Part model, mm, in its own coordinate system. A direction names the side the tool comes from. Give positions to 0.01 mm unless a question says otherwise; leave off trailing zeros. Write each loop counter-clockwise with the first axis right and the second up, starting at its lowest first coordinate (ties: lowest second). Pieces come first, ordered by that corner, then holes. Notation, with made-up numbers: M 21.5,26 L 61.5,26 A28 ccw 61.5,59 Z; hole C 75,-28.75 d4. An arc over 180 degrees is marked long. Use CSV: the item, a comma, the result in double quotes. Start each with the question number.
1. Band-saw the part on C-C, the plane z = 0.2. Count the separate pieces of the cut face and the enclosed holes in it, then the cut area to 3 significant figures.
2. 3-axis set-ups, long thin cutter, end or side, ignore diameter. For faces 1 (the face through (388.624, -9.204, -0.021)), 2 (the face through (-388.974, -8.598, -0.021)), 3 (the face through (-216.72, -306.95, -0.02)): which of +Z, -Z, +X, -X, +Y, -Y reach the whole face in a straight line?
3. Band-saw the part on B-B, the plane y = 27. List the corners of the cut face in (x, z).
4. Band-saw the part on A-A, the plane x = -63.5. List the corners of the cut face in (y, z), then the cut area to 3 significant figures.
5. Mould opens along Y. For faces 4 (the face through (216.31, -307.66, -0.02)), 5 (the face through (-378.7, 54.89, -0.02)), 6 (the face through (-324.137, 149.399, -0.021)) say: pulls with the +Y half, pulls with the -Y half, needs draft (parallel to the pull), parting line crosses it, or undercut.
6. Drill centre lines: line 1 along X through (y, z) = (112, 1.3); line 2 along X through (y, z) = (-54.5, 0.55); line 3 along Y through (x, z) = (7.5, -0.55). Where is each one in solid material? Low to high. Write a range as from..to.
7. Drop flat-ended pins along their axis: pin 1 Ø1 at (x, z) = (103.5, 1) entering from -Y; pin 2 Ø1.5 at (y, z) = (-341.5, 0) entering from +X; pin 3 Ø8 at (x, y) = (-379.31, -43.84) entering from -Z; pin 4 Ø1.5 at (y, z) = (-126, 1) entering from +X. Give the stop position or say it passes through.
from build123d import *

# Parameters (mm, degrees)
SKETCH_1_R              = 3
EXTRUDE_1_DEPTH         = 1.5
SHEET_START             = -1.5
SHEET_METAL_1_OUTLINE_R = 3
SHEET_METAL_1_DEPTH     = 1.5


# Read off the part's stored shape, not the designer's step: Преобразовать-Твердое тело1
with BuildPart() as part:
    # Sketch 1 → Бобышка-Вытянуть1 (new body)
    with BuildSketch(Plane.XY):
        with BuildLine():
            Line((201.732050808, -332.910161514), (231.299038106, -281.698637287))
            Line((231.299038106, -281.698637287), (247.320508076, -290.948637287))
            Line((247.320508076, -290.948637287), (257.320508076, -273.628129211))
            Line((257.320508076, -273.628129211), (241.299038106, -264.378129211))
            Line((241.299038106, -264.378129211), (366.299038106, -47.871778265))
            Line((366.299038106, -47.871778265), (382.320508076, -57.121778265))
            Line((382.320508076, -57.121778265), (392.320508076, -39.801270189))
            Line((392.320508076, -39.801270189), (376.299038106, -30.551270189))
            Line((376.299038106, -30.551270189), (401.299038106, 12.75))
            ThreePointArc((401.299038106, 12.75), (401.700961894, 14.25), (401.299038106, 15.75))
            Line((401.299038106, 15.75), (356.732050808, 92.942286341))
            Line((356.732050808, 92.942286341), (374.052558883, 102.942286341))
            Line((374.052558883, 102.942286341), (364.052558883, 120.262794416))
            Line((364.052558883, 120.262794416), (346.732050808, 110.262794416))
            Line((346.732050808, 110.262794416), (302.165063509, 187.455080757))
            Line((302.165063509, 187.455080757), (-302.165063509, 187.455080757))
            Line((-302.165063509, 187.455080757), (-346.732050808, 110.262794416))
            Line((-346.732050808, 110.262794416), (-364.052558883, 120.262794416))
            Line((-364.052558883, 120.262794416), (-374.052558883, 102.942286341))
            Line((-374.052558883, 102.942286341), (-356.732050808, 92.942286341))
            Line((-356.732050808, 92.942286341), (-401.299038106, 15.75))
            ThreePointArc((-401.299038106, 15.75), (-401.700961894, 14.25), (-401.299038106, 12.75))
            Line((-401.299038106, 12.75), (-376.299038106, -30.551270189))
            Line((-376.299038106, -30.551270189), (-392.320508076, -39.801270189))
            Line((-392.320508076, -39.801270189), (-382.320508076, -57.121778265))
            Line((-382.320508076, -57.121778265), (-366.299038106, -47.871778265))
            Line((-366.299038106, -47.871778265), (-241.299038106, -264.378129211))
            Line((-241.299038106, -264.378129211), (-257.320508076, -273.628129211))
            Line((-257.320508076, -273.628129211), (-247.320508076, -290.948637287))
            Line((-247.320508076, -290.948637287), (-231.299038106, -281.698637287))
            Line((-231.299038106, -281.698637287), (-201.732050808, -332.910161514))
            ThreePointArc((-201.732050808, -332.910161514), (-200.633974596, -334.008237725), (-199.133974596, -334.410161514))
            Line((-199.133974596, -334.410161514), (-149.133974596, -334.410161514))
            Line((-149.133974596, -334.410161514), (-149.133974596, -352.910161514))
            Line((-149.133974596, -352.910161514), (-129.133974596, -352.910161514))
            Line((-129.133974596, -352.910161514), (-129.133974596, -334.410161514))
            Line((-129.133974596, -334.410161514), (129.133974596, -334.410161514))
            Line((129.133974596, -334.410161514), (129.133974596, -352.910161514))
            Line((129.133974596, -352.910161514), (149.133974596, -352.910161514))
            Line((149.133974596, -352.910161514), (149.133974596, -334.410161514))
            Line((149.133974596, -334.410161514), (199.133974596, -334.410161514))
            ThreePointArc((199.133974596, -334.410161514), (200.633974596, -334.008237725), (201.732050808, -332.910161514))
        make_face()
        with Locations((244.309773091, -277.663383249)):
            Circle(SKETCH_1_R, mode=Mode.SUBTRACT)
        with Locations((379.309773091, -43.836524227)):
            Circle(SKETCH_1_R, mode=Mode.SUBTRACT)
        with Locations((139.133974596, -343.660161514)):
            Circle(SKETCH_1_R, mode=Mode.SUBTRACT)
        with Locations((-139.133974596, -343.660161514)):
            Circle(SKETCH_1_R, mode=Mode.SUBTRACT)
        with Locations((-244.309773091, -277.663383249)):
            Circle(SKETCH_1_R, mode=Mode.SUBTRACT)
        with Locations((-379.309773091, -43.836524227)):
            Circle(SKETCH_1_R, mode=Mode.SUBTRACT)
        with Locations((300, 10)):
            Circle(SKETCH_1_R, mode=Mode.SUBTRACT)
        with Locations((-300, 10)):
            Circle(SKETCH_1_R, mode=Mode.SUBTRACT)
        with Locations((-360.392304845, 106.602540379)):
            Circle(SKETCH_1_R, mode=Mode.SUBTRACT)
        with Locations((360.392304845, 106.602540379)):
            Circle(SKETCH_1_R, mode=Mode.SUBTRACT)
    extrude(amount=EXTRUDE_1_DEPTH)

    # Sheet Metal 1 outline → Sheet Metal 1 (add)
    with BuildSketch(Plane.XY.offset(SHEET_START)):
        with BuildLine():
            Line((-199.133974596, -334.410161514), (-149.133974596, -334.410161514))
            Line((-149.133974596, -334.410161514), (-149.133974596, -352.910161514))
            Line((-149.133974596, -352.910161514), (-129.133974596, -352.910161514))
            Line((-129.133974596, -352.910161514), (-129.133974596, -334.410161514))
            Line((-129.133974596, -334.410161514), (129.133974596, -334.410161514))
            Line((129.133974596, -334.410161514), (129.133974596, -352.910161514))
            Line((129.133974596, -352.910161514), (149.133974596, -352.910161514))
            Line((149.133974596, -352.910161514), (149.133974596, -334.410161514))
            Line((149.133974596, -334.410161514), (199.133974596, -334.410161514))
            ThreePointArc((199.133974596, -334.410161514), (200.633974596, -334.008237725), (201.732050808, -332.910161514))
            Line((201.732050808, -332.910161514), (231.299038106, -281.698637287))
            Line((231.299038106, -281.698637287), (247.320508076, -290.948637287))
            Line((247.320508076, -290.948637287), (257.320508076, -273.628129211))
            Line((257.320508076, -273.628129211), (241.299038106, -264.378129211))
            Line((241.299038106, -264.378129211), (366.299038106, -47.871778265))
            Line((366.299038106, -47.871778265), (382.320508076, -57.121778265))
            Line((382.320508076, -57.121778265), (392.320508076, -39.801270189))
            Line((392.320508076, -39.801270189), (376.299038106, -30.551270189))
            Line((376.299038106, -30.551270189), (401.299038106, 12.75))
            ThreePointArc((401.299038106, 12.75), (401.700961894, 14.25), (401.299038106, 15.75))
            Line((401.299038106, 15.75), (356.732050808, 92.942286341))
            Line((356.732050808, 92.942286341), (374.052558883, 102.942286341))
            Line((374.052558883, 102.942286341), (364.052558883, 120.262794416))
            Line((364.052558883, 120.262794416), (346.732050808, 110.262794416))
            Line((346.732050808, 110.262794416), (302.165063509, 187.455080757))
            Line((302.165063509, 187.455080757), (-302.165063509, 187.455080757))
            Line((-302.165063509, 187.455080757), (-346.732050808, 110.262794416))
            Line((-346.732050808, 110.262794416), (-364.052558883, 120.262794416))
            Line((-364.052558883, 120.262794416), (-374.052558883, 102.942286341))
            Line((-374.052558883, 102.942286341), (-356.732050808, 92.942286341))
            Line((-356.732050808, 92.942286341), (-401.299038106, 15.75))
            ThreePointArc((-401.299038106, 15.75), (-401.700961894, 14.25), (-401.299038106, 12.75))
            Line((-401.299038106, 12.75), (-376.299038106, -30.551270189))
            Line((-376.299038106, -30.551270189), (-392.320508076, -39.801270189))
            Line((-392.320508076, -39.801270189), (-382.320508076, -57.121778265))
            Line((-382.320508076, -57.121778265), (-366.299038106, -47.871778265))
            Line((-366.299038106, -47.871778265), (-241.299038106, -264.378129211))
            Line((-241.299038106, -264.378129211), (-257.320508076, -273.628129211))
            Line((-257.320508076, -273.628129211), (-247.320508076, -290.948637287))
            Line((-247.320508076, -290.948637287), (-231.299038106, -281.698637287))
            Line((-231.299038106, -281.698637287), (-201.732050808, -332.910161514))
            ThreePointArc((-201.732050808, -332.910161514), (-200.633974596, -334.008237725), (-199.133974596, -334.410161514))
        make_face()
        with Locations((-244.309773091, -277.663383249)):
            Circle(SHEET_METAL_1_OUTLINE_R, mode=Mode.SUBTRACT)
        with Locations((-139.133974596, -343.660161514)):
            Circle(SHEET_METAL_1_OUTLINE_R, mode=Mode.SUBTRACT)
        with Locations((139.133974596, -343.660161514)):
            Circle(SHEET_METAL_1_OUTLINE_R, mode=Mode.SUBTRACT)
        with Locations((244.309773091, -277.663383249)):
            Circle(SHEET_METAL_1_OUTLINE_R, mode=Mode.SUBTRACT)
        with Locations((-379.309773091, -43.836524227)):
            Circle(SHEET_METAL_1_OUTLINE_R, mode=Mode.SUBTRACT)
        with Locations((-300, 10)):
            Circle(SHEET_METAL_1_OUTLINE_R, mode=Mode.SUBTRACT)
        with Locations((-360.392304845, 106.602540379)):
            Circle(SHEET_METAL_1_OUTLINE_R, mode=Mode.SUBTRACT)
        with Locations((379.309773091, -43.836524227)):
            Circle(SHEET_METAL_1_OUTLINE_R, mode=Mode.SUBTRACT)
        with Locations((300, 10)):
            Circle(SHEET_METAL_1_OUTLINE_R, mode=Mode.SUBTRACT)
        with Locations((360.392304845, 106.602540379)):
            Circle(SHEET_METAL_1_OUTLINE_R, mode=Mode.SUBTRACT)
    extrude(amount=SHEET_METAL_1_DEPTH)


solid = part.part
Output:
1,separate pieces,"1"
1,enclosed holes,"10"
1,area,"335,000 mm²"
2,face 1,"+Z, -Z, +X"
2,face 2,"+Z, -Z, -X"
2,face 3,"+Z, -Z, -Y"
3,outline,"M -394.8,-1.5 L 394.8,-1.5 L 394.8,1.5 L -394.8,1.5 Z"
4,outline,"M -334.41,-1.5 L 187.46,-1.5 L 187.46,1.5 L -334.41,1.5 Z"
4,area,"1,570 mm²"
5,face 4,"pulls with the -Y half"
5,face 5,"undercut"
5,face 6,"pulls with the +Y half"
6,line 1,"x = -368.82..-349.74, -345.73..345.73, 349.74..368.82"
6,line 2,"x = -383.83..-377.78, -362.47..362.47, 377.78..383.83"
6,line 3,"y = -334.41..187.46"
7,pin 1,"stops at y = -334.41"
7,pin 2,"stops at x = 149.13"
7,pin 3,"stops at z = -1.5"
7,pin 4,"stops at x = 321.62"
